Autodesk Inventor part; units mm, degrees
ref_plane "YZ Plane" through (0, 0, 0) normal (1, 0, 0) x (0, 1, 0)
ref_plane "XZ Plane" through (0, 0, 0) normal (0, 1, 0) x (-1, 0, 0)
ref_plane "XY Plane" through (0, 0, 0) normal (0, 0, 1) x (1, 0, 0)
sketch "Sketch1" plane through (0, 0, 0) normal (0, 0, 1) x (1, 0, 0)
  line L0 (0, 0) -> (25.4, 0)
  line L1 (25.4, 0) -> (25.4, 1.5875)
  line L2 (1.5875, 50.8) -> (0, 50.8)
  line L3 (0, 50.8) -> (0, 0)
  line L4 (1.5875, 50.8) -> (1.5875, 1.5875)
  line L5 (1.5875, 1.5875) -> (25.4, 1.5875)
  dimension "d0" = 1.5875
  dimension "d1" = 1.5875
  dimension "d2" = 25.4
  dimension "d3" = 50.8
extrude "Extrusion1" add sketch "Sketch1" along normal blind 457.2
sketch "Sketch2" plane through (0, 0, 0) normal (-1, 0, 0) x (0, 0, 1)
  line L0 (457.2, 0) -> (457.2, 50.8)
  line L1 (0, 50.8) -> (457.2, 50.8)
  line L2 (0, 50.8) -> (0, 0)
  line L3 (0, 0) -> (457.2, 0)
  line L4 (19.05, 50.8) -> (19.05, 31.75)
  line L5 (19.05, 31.75) -> (431.8, 31.75)
  circle A0 centre (12.7, 44.45) radius 3.175
  arc A1 (19.05, 44.45) -> (12.7, 50.8) centre (12.7, 44.45) ccw
  circle A2 centre (444.5, 31.75) radius 11.1125 construction
  line L6 (431.8, 31.75) -> (431.8, 41.275)
  circle A3 centre (444.5, 31.75) radius 2.54
  line L7 (431.8, 41.275) -> (457.2, 41.275)
  circle A4 centre (277.8125, 12.7) radius 11.1125 construction
  circle A5 centre (277.8125, 12.7) radius 2.54
  line L8 (266.7, 0) -> (266.7, -29.1939)
  dimension "d6" = 19.05
  dimension "d7" = 19.05
  dimension "d8" = 6.35
  dimension "d9" = 12.7
  dimension "d10" = 6.35
  dimension "d13" = 22.225
  dimension "d14" = 25.4
  dimension "d15" = 5.08
  dimension "d16" = 31.75
  dimension "d17" = 12.7
  dimension "d18" = 9.525
  dimension "d19" = 12.7
  dimension "d27" = 190.5
extrude "Extrusion2" cut sketch "Sketch2" against normal through all contours L7 L6 L5 L4 L1 L0 | L4 A1 L1 | A0 | A3 | A5
sketch "Sketch3" plane through (0, 0, 0) normal (0, -1, 0) x (1, 0, 0)
  line L0 (0, 0) -> (0, 457.2)
  line L1 (0, 0) -> (25.4, 0)
  line L2 (25.4, 0) -> (25.4, 457.2)
  circle A0 centre (19.05, 79.375) radius 1.5875
  circle A1 centre (6.35, 92.075) radius 1.5875
  line L3 (0, 265.1125) -> (25.4, 265.1125) construction
  circle A2 centre (19.05, 450.85) radius 1.5875
  circle A3 centre (6.35, 438.15) radius 1.5875
  line L4 (25.4, 457.2) -> (0, 457.2)
  line L5 (25.4, 0) -> (25.4, 457.2)
  line L6 (0, 0) -> (0, 457.2)
  dimension "d20" = 3.175
  dimension "d21" = 6.35
  dimension "d22" = 6.35
  dimension "d24" = 79.375
  dimension "d28" = 6.35
  dimension "d29" = 6.35
  dimension "d30" = 12.7
extrude "Extrusion3" cut sketch "Sketch3" against normal through all contours A0 | A1 | A2 | A3
equation "\"d0\" = d1"
properties part number "8 ball top roller L frame"
Can you work these out from the model? Positions are in its coordinate system, mm. A direction names the side the tool comes from. Give positions to 0.01 mm unless a question says otherwise; leave off trailing zeros. Loops run counter-clockwise (first coordinate to the right, second up) from the corner with the lowest first, then second, coordinate; pieces in that order, holes last. Notation, with made-up numbers: M -20,-13 L -13,-13 A14 cw -13,4 Z; hole C 68,83.5 d7. An arc over 180 degrees is marked long. Use one line per item in the form item = value. Start each with the question number.
(1) Please list where these lines run through material, in increasing order: line 1 (Z direction, x = 19.05, y = 0.45); line 2 (X direction, y = 0.4, z = 438.15); line 3 (Y direction, x = 0.8, z = 444.5) (3 decimals).
(2) I want a section at A-A, the plane z = 293.5. Write out the boundary of the cut face in (x, y), and give its area (3 significant figures).
(3) On a 3-axis mill with a long thin cutter (end or side, diameter ignored), from which of +Z, -Z, +X, -X, +Y, -Y can I reach the whole of each face in a straight line? I mean faces 1 (the flat face through (13, 1.588, 225)), 2 (the flat face through (13, 0, 225)). Say none if no direction works.
(4) I'm going to push flat-ended pins straight in: P1, Ø6, axis at y = 7, z = 316.5, coming from the +X side; P2, Ø2.5, axis at x = 6.35, z = 92.075, coming from the -Y side; P3, Ø12, axis at x = 18, z = 265.5, coming from the +Y side; P4, Ø0.5, axis at x = 0.5, z = 307.5, coming from the +Y side. Where does each tip first touch, or does it pass through?
Worked out:
q1.line_1 = 0 to 77.79, 80.96 to 449.26, 452.44 to 457.2
q1.line_2 = 0 to 4.76, 7.94 to 25.4
q1.line_3 = 0 to 29.21, 34.29 to 41.275
q2.outline = M 0,0 L 25.4,0 L 25.4,1.59 L 1.59,1.59 L 1.59,31.75 L 0,31.75 Z
q2.area = 88.2 mm²
q3.face_1 = +Z, -Z, +X, +Y
q3.face_2 = +Z, -Z, +X, -X, -Y
q4.P1 = 1.59
q4.P2 = through
q4.P3 = 1.59
q4.P4 = 31.75
